For this review, take the finished solid that the model builds, in its own axes (mm). Face numbers are marked on the shaded views. Round coordinates to 2 decimals unless told otherwise and drop trailing zeros. Loops run counter-clockwise (first coordinate to the right, second up) from the corner with the lowest first, then second, coordinate; pieces in that order, holes last.
1. Draft analysis for pull direction Y (two halves, no side actions). For the marked faces 1 and 2, state which applies: released by +Y, released by -Y, zero draft, split by the parting line, or undercut.
2. Consider section B-B on y = -4. State how many separate pieces and enclosed holes the cut face has, then the cut area to 3 significant figures.
3. Consider section A-A on z = 25. State the section outline as (x, y) points, then the cut area to 3 significant figures.
4. To check wall thickness, follow line 1 along Z through (x, y) = (-98, -11.5); line 2 along X through (y, z) = (-5.5, -10); line 3 along X through (y, z) = (-6, 72.5). State the ranges of each line that lie inside material, in increasing order.
5. Clearance check with flat-ended pins moving along their axes: pin 1 Ø8 at (x, y) = (-90.5, -6) entering from +Z; pin 2 Ø10 at (x, z) = (-27.5, 67) entering from -Y; pin 3 Ø3 at (y, z) = (-13, 62) entering from +X; pin 4 Ø8 at (y, z) = (-4.5, 93.5) entering from -X. State where each tip first meets the part, or that it passes through.
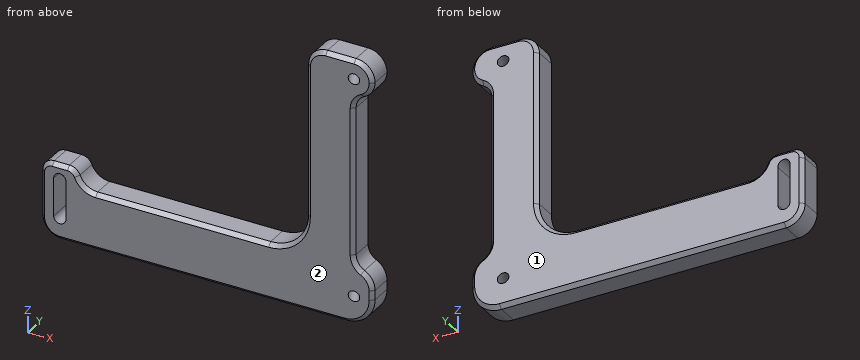
from build123d import *

# Parameters (mm, degrees)
F1_DEPTH = 15
F3_DEPTH = 20
F8_D     = 5.5
F9_R     = 8
F10_R    = 6
F11_R    = 10
F12_SIZE = 2


# Not quite as in the source:
# - ends of sketch curves that miss each other by under 0.0002 mm in the source are joined


with BuildPart() as f1:
    # F0 (on Front) → F1 (new body)
    with BuildSketch(Plane.XZ):
        with BuildLine():
            Line((-2.8333987482, 0), (-2.8333987482, 90))
            ThreePointArc((-2.8333987482, 90), (4.2344373086, 92.9306997935), (7.1616023332, 100))
            ThreePointArc((7.1616023332, 100), (4.2326701451, 107.0710678119), (-2.8383976668, 110))
            Line((-2.8383976668, 110), (-17.8333987482, 110))
            ThreePointArc((-17.8333987482, 110), (-24.9044665601, 107.0710678119), (-27.8333987482, 100))
            Line((-27.8333987482, 100), (-27.8333987482, 20))
            ThreePointArc((-27.8333987482, 20), (-33.6912631245, 5.8578643763), (-47.8333987482, 0))
            Line((-47.8333987482, 0), (-147.8333987482, 0))
            Line((-147.8333987482, 0), (-147.8333987482, 10))
            Line((-147.8333987482, 10), (-153.8333987482, 10))
            Line((-153.8333987482, 10), (-161.8333987482, 10))
            ThreePointArc((-161.8333987482, 10), (-166.0760394353, 8.2426406871), (-167.8333987482, 4))
            Line((-167.8333987482, 4), (-167.8333987482, -20))
            ThreePointArc((-167.8333987482, -20), (-164.9044665601, -27.0710678119), (-157.8333987482, -30))
            Line((-157.8333987482, -30), (-7.8333987482, -30))
            ThreePointArc((-7.8333987482, -30), (2.7732029696, -25.6066017178), (7.1666012518, -15))
            Line((7.1666012518, -15), (7.1666012518, -10))
            ThreePointArc((7.1666012518, -10), (4.2376690637, -2.9289321881), (-2.8333987482, 0))
        make_face()
    extrude(amount=F1_DEPTH)

    # F2 (on face) → F3 (cut)
    with BuildSketch(Plane.XZ.offset(15)):
        with BuildLine():
            Line((-154.5833987482, -18), (-154.5833987482, 2))
            ThreePointArc((-154.5833987482, 2), (-157.8333987482, 5.25), (-161.0833987482, 2))
            Line((-161.0833987482, 2), (-161.0833987482, -18))
            ThreePointArc((-161.0833987482, -18), (-157.8333987482, -21.25), (-154.5833987482, -18))
        make_face()
    extrude(amount=-F3_DEPTH, mode=Mode.SUBTRACT)

    # F8 (through all)
    with Locations(Plane(origin=(-9.7913406688, 20.9975978253, 0), x_dir=(-0.906307787, -0.4226182617, 0), z_dir=(-0.4226182617, 0.906307787, 0))):
        with Locations((8.9072052754, 100), (8.9072052754, -15)):
            Hole(F8_D / 2)

    # F9
    f9_edges = [f1.edges().sort_by_distance(p)[0] for p in [
        (-2.833399, -7.5, 0),
        (-2.833399, -7.5, 90),
    ]]
    fillet(f9_edges, radius=F9_R)

    # F10
    f10_edges = [f1.edges().sort_by_distance(p)[0] for p in [
        (-147.833399, -7.5, 10),
    ]]
    fillet(f10_edges, radius=F10_R)

    # F11
    f11_edges = [f1.edges().sort_by_distance(p)[0] for p in [
        (-147.833399, -7.5, 0),
    ]]
    fillet(f11_edges, radius=F11_R)

    # F12
    f12_edges = [f1.edges().sort_by_distance(p)[0] for p in [
        (-93.4172, -15, 0),
        (-93.4172, 0, 0),
        (-150.479297, 0, 8.974937),
        (-144.591172, 0, 1.708438),
        (-157.833399, 0, 10),
        (-166.076039, 0, 8.242641),
        (-33.691263, 0, 5.857864),
        (-167.833399, 0, -8),
        (-27.833399, 0, 60),
        (-164.904467, 0, -27.071068),
        (-24.904467, 0, 107.071068),
        (-82.833399, 0, -30),
        (-10.335898, 0, 110),
        (2.773203, 0, -25.606602),
        (4.23267, 0, 107.071068),
        (7.166601, 0, -12.5),
        (5.660785, 0, 94.730854),
        (5.664967, 0, -4.729537),
        (-1.632745, 0, 88.093281),
        (-1.632091, 0, 1.908145),
        (-2.833399, 0, 45.00124),
        (-150.479297, -15, 8.974937),
        (-144.591172, -15, 1.708438),
        (-157.833399, -15, 10),
        (-166.076039, -15, 8.242641),
        (-33.691263, -15, 5.857864),
        (-167.833399, -15, -8),
        (-27.833399, -15, 60),
        (-164.904467, -15, -27.071068),
        (-24.904467, -15, 107.071068),
        (-82.833399, -15, -30),
        (-10.335898, -15, 110),
        (2.773203, -15, -25.606602),
        (4.23267, -15, 107.071068),
        (7.166601, -15, -12.5),
        (5.660785, -15, 94.730854),
        (5.664967, -15, -4.729537),
        (-1.632745, -15, 88.093281),
        (-1.632091, -15, 1.908145),
        (-2.833399, -15, 45.00124),
    ]]
    chamfer(f12_edges, length=F12_SIZE)


solid = f1.part
Resolved:
1. face 1: released by +Y
1. face 2: released by -Y
2. separate pieces: 1
2. enclosed holes: 3
2. area: 8,120 mm2
3. outline: (-27.83, -13) - (-25.83, -15) - (-4.83, -15) - (-2.83, -13) - (-2.83, -2) - (-4.83, 0) - (-25.83, 0) - (-27.83, -2) - close
3. area: 367 mm2
4. line 1: z = -30 to 0
4. line 2: x = -167.83 to -161.08, -154.58 to 7.17
4. line 3: x = -27.83 to -2.83
5. pin 1: stops at z = 0
5. pin 2: stops at y = -15
5. pin 3: stops at x = -2.83
5. pin 4: stops at x = -27.83
